The listing builds one solid part. Answer for the finished solid, in the listing's coordinates (mm). A direction names the side the tool comes from. Round coordinates to 2 decimals unless told otherwise and drop trailing zeros. Write each loop counter-clockwise with the first axis right and the second up, starting at its lowest first coordinate (ties: lowest second). Pieces come first, ordered by that corner, then holes. Notation, with made-up numbers: (10, 29) -> (66, 29) arc R19 ccw to (66, 58) -> close; hole circle Ø5 at (75, -22.5). An arc over 180 degrees is marked (long way). Write each question's results on one line, items separated by ' | '. Start each with the question number.
```python
from build123d import *

# Parameters (mm, degrees)
F0_R     = 38.1
F0_R_2   = 31.75
F1_DEPTH = 25.4
F0_R_3   = 25.4
F2_DEPTH = 31.75
F0_R_4   = 3.175
F3_DEPTH = 19.05


with BuildPart() as f1:
    # F0 (on Front) → F1 (new body)
    with BuildSketch(Plane.XZ):
        Circle(F0_R)
        Circle(F0_R_2, mode=Mode.SUBTRACT)
    extrude(amount=F1_DEPTH)

    # F0 (on Front) → F2 (join)
    with BuildSketch(Plane.XZ):
        Circle(F0_R_2)
        Circle(F0_R_3, mode=Mode.SUBTRACT)
    extrude(amount=F2_DEPTH)

    # F0 (on Front) → F3 (join)
    with BuildSketch(Plane.XZ):
        Circle(F0_R_3)
        with Locations((0, -19.05)):
            Circle(F0_R_4, mode=Mode.SUBTRACT)
        with Locations((-19.05, 0)):
            Circle(F0_R_4, mode=Mode.SUBTRACT)
        Circle(F0_R_4, mode=Mode.SUBTRACT)
        with Locations((19.05, 0)):
            Circle(F0_R_4, mode=Mode.SUBTRACT)
        with Locations((0, 19.05)):
            Circle(F0_R_4, mode=Mode.SUBTRACT)
    extrude(amount=F3_DEPTH)


solid = f1.part
```
Q1. For faces 1 (the flat face through (5, -19.05, 0)), 2 (the cylindrical face through (-0.69, -9.39, -3.1)), determine the directions among +Z, -Z, +X, -X, +Y, -Y from which every point of the face is accessible in a straight line to the end or side of a thin tool.
Q2. The part is cut by section C-C, the plane z = 18. Write down the section's boundary in (x, y).
Q3. Determine the mould class of faces 3 (the flat face through (-9, -25.4, 31)), 4 (the cylindrical face through (-5.506, -25.311, -24.796)), 5 (the cylindrical face through (-30.235, -12.522, -23.183)) for opening direction Z: pulls with the +Z half, pulls with the -Z half, needs draft (parallel to the pull), parting line crosses it, or undercut.
Q4. Find the intervals of material crossed by line 1 (Z direction, x = 0, y = -12.5) (3 decimals); line 2 (Y direction, x = 34, z = 12.5); line 3 (Z direction, x = 0, y = -26), in increasing order.
Q5. The part is cut by section D-D, the plane y = -26.5. Write down the section's boundary in (x, z), then the cut area to 3 significant figures.
Q6. The part is cut by section A-A, the plane z = 0. Write down the section's boundary in (x, y) (3 decimals), then the cut area to 3 significant figures.
Q7. Each of these flat-tipped pins is pushed along its axis until it touches: pin 1 (12 mm diameter, centred on x = 16.5, y = -15, fed in from -Z); pin 2 (15 mm diameter, centred on x = -2.5, z = 2.5, fed in from -Y); pin 3 (8 mm diameter, centred on x = -9, y = -21, fed in from +Z). Where does it stop, or does it pass through?
Q8. The part is cut by section B-B, the plane x = -19.05. Write down the section's boundary in (y, z) (3 decimals).
Answers follow:
1) face 1: -Y | face 2: +Y, -Y
2) outline: (-33.58, -25.4) -> (-26.15, -25.4) -> (-26.15, -31.75) -> (-17.92, -31.75) -> (-17.92, -19.05) -> (-3, -19.05) -> (-3, 0) -> (-33.58, 0) -> close; (3, -19.05) -> (17.92, -19.05) -> (17.92, -31.75) -> (26.15, -31.75) -> (26.15, -25.4) -> (33.58, -25.4) -> (33.58, 0) -> (3, 0) -> close
3) face 3: needs draft | face 4: undercut | face 5: parting line crosses it
4) line 1: -38.1 to -22.225, -15.875 to -3.175, 3.175 to 15.875, 22.225 to 38.1 | line 2: -25.4 to 0 | line 3: -31.75 to -25.4, 25.4 to 31.75
5) outline: circle Ø63.5 at (0, 0); hole circle Ø50.8 at (0, 0) | area: 1,140 mm^2
6) outline: (-38.1, -25.4) -> (-31.75, -25.4) -> (-31.75, -31.75) -> (-25.4, -31.75) -> (-25.4, -19.05) -> (-22.225, -19.05) -> (-22.225, 0) -> (-38.1, 0) -> close; (-15.875, -19.05) -> (-3.175, -19.05) -> (-3.175, 0) -> (-15.875, 0) -> close; (3.175, -19.05) -> (15.875, -19.05) -> (15.875, 0) -> (3.175, 0) -> close; (22.225, -19.05) -> (25.4, -19.05) -> (25.4, -31.75) -> (31.75, -31.75) -> (31.75, -25.4) -> (38.1, -25.4) -> (38.1, 0) -> (22.225, 0) -> close | area: 1,330 mm^2
7) pin 1: z = -36.62 | pin 2: y = -19.05 | pin 3: z = 37.77
8) outline: (-31.75, -25.4) -> (-25.4, -25.4) -> (-25.4, -32.996) -> (0, -32.996) -> (0, -3.175) -> (-19.05, -3.175) -> (-19.05, -16.801) -> (-31.75, -16.801) -> close; (-31.75, 16.801) -> (-19.05, 16.801) -> (-19.05, 3.175) -> (0, 3.175) -> (0, 32.996) -> (-25.4, 32.996) -> (-25.4, 25.4) -> (-31.75, 25.4) -> close
